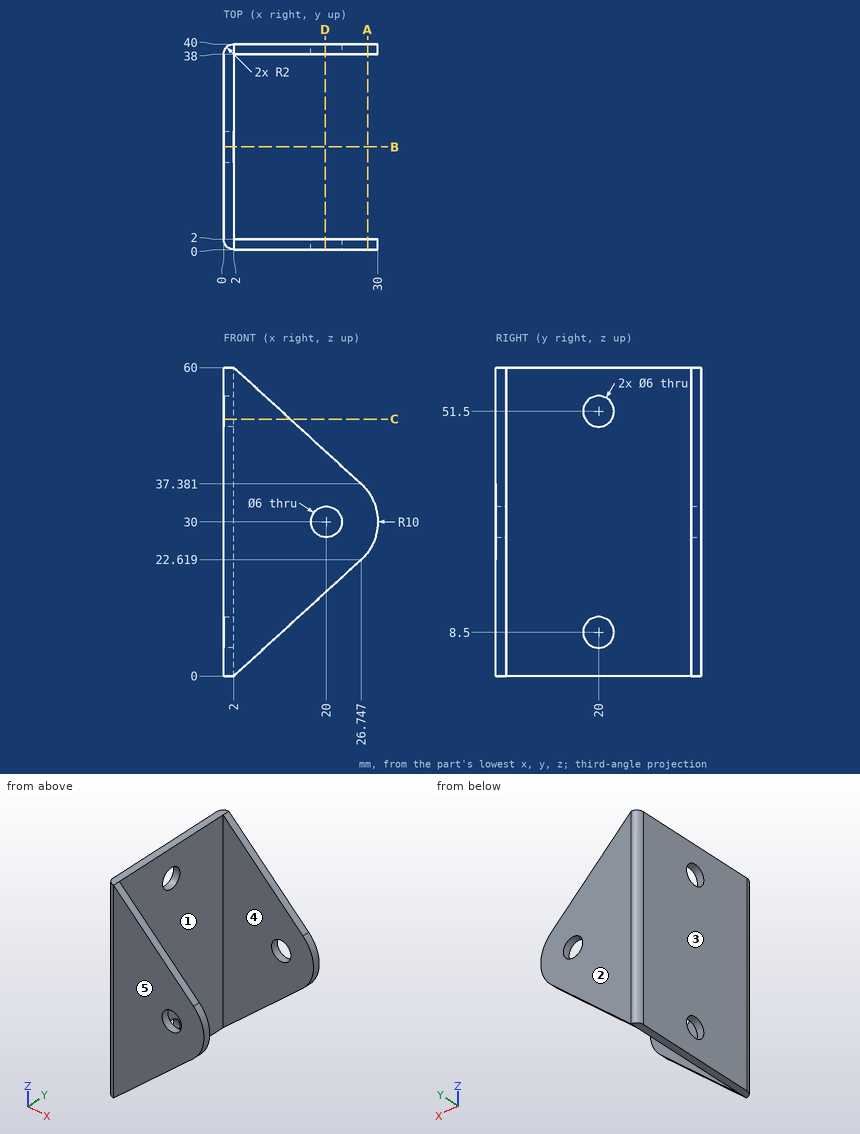
Could you check a few things on this drawing? It's one solid part, dimensions in mm from its lowest x, y, z. A direction names the side the tool comes from. Give positions to 0.01 mm unless a question says otherwise; leave off trailing zeros. Order: outer loops, then holes, each group sorted by start corner. A loop starts at its lowest first (then second) coordinate and runs counter-clockwise, first axis right, second up. Notation, with made-up numbers: (4.5, 48) -> (30.5, 48) arc R30 ccw to (30.5, 80) -> close; hole circle Ø4 at (-25.5, 73). An arc over 180 degrees is marked (long way). Answer in a Markdown table with one row per item. Add a question column.
Item 1: Imagine slicing it at A-A (x = 28). List the corners of the cut face in (y, z) for me.
Item 2: We'd pull the mould along Y, two halves only. Please class the marked faces 3, 4 and 5: pulls with the +Y half, pulls with the -Y half, needs draft (parallel to the pull), parting line crosses it, or undercut.
Item 3: Please list where these lines run through material, in increasing order: probe 1 along Y at (x, z) = (21.25, 35.5); probe 2 along X at (y, z) = (22, 27); probe 3 along Y at (x, z) = (0.95, 51.5).
Item 4: Imagine slicing it at D-D (x = 19.75). List the corners of the cut face in (y, z) for me.
Item 5: Imagine slicing it at C-C (z = 50). List the corners of the cut face in (x, y) for me, and give its area (3 significant figures).
Item 6: For the marked faces 1 and 2, which set-ups out of +Z, -Z, +X, -X, +Y, -Y let a thin tool reach every point of the face, with its end or its side?
Item 7: I'm going to push flat-ended pins straight in: P1, Ø10, axis at y = 28, z = 8.5, coming from the +X side; P2, Ø10, axis at x = 17, y = 6.5, coming from the +Z side. Where does each tip first touch, or does it pass through?
Item 8: Imagine slicing it at B-B (y = 20). List the corners of the cut face in (x, z) for me.
Result:
| question | item | result |
|---|---|---|
| 1 | outline | (0, 24) -> (2, 24) -> (2, 36) -> (0, 36) -> close; (38, 24) -> (40, 24) -> (40, 36) -> (38, 36) -> close |
| 2 | face 3 | needs draft |
| 2 | face 4 | undercut |
| 2 | face 5 | pulls with the -Y half |
| 3 | probe 1 | 0 to 2, 38 to 40 |
| 3 | probe 2 | 0 to 2 |
| 3 | probe 3 | 0.3 to 17, 23 to 39.7 |
| 4 | outline | (0, 16.22) -> (2, 16.22) -> (2, 27.01) -> (0, 27.01) -> close; (0, 32.99) -> (2, 32.99) -> (2, 43.78) -> (0, 43.78) -> close; (38, 16.22) -> (40, 16.22) -> (40, 27.01) -> (38, 27.01) -> close; (38, 32.99) -> (40, 32.99) -> (40, 43.78) -> (38, 43.78) -> close |
| 5 | outline | (0, 2) arc R2 ccw to (2, 0) -> (12.94, 0) -> (12.94, 2) -> (2, 2) -> (2, 17.4) -> (0, 17.4) -> close; (0, 22.6) -> (2, 22.6) -> (2, 38) -> (12.94, 38) -> (12.94, 40) -> (2, 40) arc R2 ccw to (0, 38) -> close |
| 5 | area | 112 mm2 |
| 6 | face 1 | +Z, -Z, +X |
| 6 | face 2 | +Z, -Z, +X, -X, +Y |
| 7 | P1 | x = 2 |
| 7 | P2 | z = 48.28 |
| 8 | outline | (0, 0) -> (2, 0) -> (2, 5.5) -> (0, 5.5) -> close; (0, 11.5) -> (2, 11.5) -> (2, 48.5) -> (0, 48.5) -> close; (0, 54.5) -> (2, 54.5) -> (2, 60) -> (0, 60) -> close |
